Solid Edge part; units mm, degrees
sketch "Sketch1" plane through (0, 0, 0) normal (1, 0, 0) x (0, 1, 0)
  line L0 (80, 0) -> (80, 20)
  line L1 (80, 20) -> (0, 20)
  line L2 (0, 20) -> (0, 0)
  line L3 (0, 0) -> (80, 0)
extrude "Protrusion1" add sketch "Sketch1" against normal blind 10
sketch "Sketch2" plane through (0, 32.5, 7.5) normal (1, 0, 0) x (0, 1, 0)
  circle A0 centre (7.5, 2.5) radius 7.5
extrude "Cutout1" cut sketch "Sketch2" against normal through all
hole "Bohrung_1" at (-5, 40, 20) direction (0, 0, -1) diameter 4.917 end up to next
Build history of the part. All positions in model axes, mm. Round coordinates to 2 decimals unless told otherwise and drop trailing zeros. Order: outer loops, then holes, each group sorted by start corner. A loop starts at its lowest first (then second) coordinate and runs counter-clockwise, first axis right, second up. Notation, with made-up numbers: (0.5, -7) -> (41.5, -7) arc R18 cw to (41.5, 9) -> close; hole circle Ø7 at (45, 13.25). An arc over 180 degrees is marked (long way). Answer in a Markdown table with one row per item.
1) Band-saw the part on B-B on x = -5. Give the cut face in (y, z), and give its area (3 significant figures).
Values:
| item | result |
|---|---|
| outline | (0, 0) -> (80, 0) -> (80, 20) -> (42.46, 20) -> (42.46, 17.09) arc R7.5 cw (long way) to (37.54, 17.09) -> (37.54, 20) -> (0, 20) -> close |
| area | 1,410 mm2 |
2) Band-saw the part on C-C on x = -8.5. Give the cut face in (y, z).
Values:
| item | result |
|---|---|
| outline | (0, 0) -> (80, 0) -> (80, 20) -> (0, 20) -> close; hole circle Ø15 at (40, 10) |
3) Mould opens along X. For faces 1 (the cylindrical face through (-7.2, 38.9, 18.6)), 2 (the flat face through (-2, 41, 20)), 3 (the flat face through (-10, 39, 19)), 4 (the flat face through (0, 39, 19)) say: released by +X, released by -X, zero draft, split by the parting line, or undercut.
Values:
| item | result |
|---|---|
| face 1 | undercut |
| face 2 | zero draft |
| face 3 | released by -X |
| face 4 | released by +X |
4) Pin check, flat tips, straight feed: P1, Ø9, axis at y = 40, z = 10, coming from the +X side; P2, Ø4.5, axis at x = -5, y = 40, coming from the +Z side. Stop position of each tip, or through.
Values:
| item | result |
|---|---|
| P1 | through |
| P2 | z = 2.85 |
5) Wall check: L1, parallel to X at y = 40, z = 17.9; L2, parallel to Z at x = -7.5, y = 40; L3, parallel to Y at x = -5, z = 19.15. Give the ranges that are in metal, low to high.
Values:
| item | result |
|---|---|
| L1 | -10 to -7.46, -2.54 to 0 |
| L2 | 0 to 2.5, 17.5 to 20 |
| L3 | 0 to 37.54, 42.46 to 80 |
6) Band-saw the part on A-A on y = 40. Give the cut face in (x, z), and give its area (3 significant figures).
Values:
| item | result |
|---|---|
| outline | (-10, 0) -> (0, 0) -> (0, 2.5) -> (-10, 2.5) -> close; (-10, 17.5) -> (-7.46, 17.5) -> (-7.46, 20) -> (-10, 20) -> close; (-2.54, 17.5) -> (0, 17.5) -> (0, 20) -> (-2.54, 20) -> close |
| area | 37.7 mm2 |
